Autodesk Inventor part; units mm, degrees
ref_plane "YZ Plane" through (0, 0, 0) normal (1, 0, 0) x (0, 1, 0)
ref_plane "XZ Plane" through (0, 0, 0) normal (0, 1, 0) x (-1, 0, 0)
ref_plane "XY Plane" through (0, 0, 0) normal (0, 0, 1) x (1, 0, 0)
sketch "Skizze1" plane through (0, 0, 0) normal (1, 0, 0) x (0, 1, 0)
  line L0 (-20, 20) -> (20, 20)
  line L1 (20, 20) -> (20, -20)
  line L2 (20, -20) -> (-20, -20)
  line L3 (-20, -20) -> (-20, 20)
  line L4 (-20, 20) -> (20, -20) construction
  line L5 (20, 20) -> (-20, -20) construction
  line L6 (-18, 18) -> (18, 18)
  line L7 (18, 18) -> (18, -18)
  line L8 (18, -18) -> (-18, -18)
  line L9 (-18, -18) -> (-18, 18)
  line L10 (-18, 18) -> (18, -18) construction
  line L11 (18, 18) -> (-18, -18) construction
  point P0 (0, 0)
  dimension "d0" = 40
  dimension "d1" = 40
  dimension "d2" = 36
  dimension "d3" = 36
extrude "Extrusion1" add sketch "Skizze1" along normal blind 1250
sketch "Skizze2" plane through (0, -20, 20) normal (0, 0, 1) x (1, 0, 0)
  circle A0 centre (20, 20) radius 5.25
  line L0 (1250, 2) -> (1250, 38)
  circle A1 centre (1150, 20) radius 5.25
  point P0 (0, 20)
  dimension "d7" = 10.5
  dimension "d11" = 10.5
extrude "Extrusion2" cut sketch "Skizze2" against normal blind 1250
sketch "Skizze3" plane through (0, 20, 20) normal (0, 1, 0) x (1, 0, 0)
  line L0 (0, 20) -> (110, 20)
  circle A0 centre (110, 20) radius 3.2
  dimension "d14" = 110
  dimension "d15" = 6.4
extrude "Extrusion3" cut sketch "Skizze3" against normal blind 5
sketch "Skizze4" plane through (0, -20, -20) normal (0, -1, 0) x (1, 0, 0)
  circle A0 centre (110, 20) radius 3.2
  line L0 (0, 20) -> (110, 20)
  circle A1 centre (110, 20) radius 5.5
  dimension "d18" = 110
  dimension "d19" = 11
extrude "Extrusion4" cut sketch "Skizze4" against normal blind 5 contours A0 | A1
fillet "Rundung1" radius 1 4 edges at (625, 20, -20) (625, -20, -20) (625, -20, 20) (625, 20, 20)
fillet "Rundung2" radius 0.5 4 edges at (625, -18, 18) (625, -18, -18) (625, 18, -18) (625, 18, 18)
sketch "Skizze6" plane through (0, -19, -20) normal (0, 0, -1) x (-1, 0, 0)
  line L0 (0, 19) -> (-500, 19)
  circle A0 centre (-500, 19) radius 14
  dimension "d28" = 500
  dimension "d29" = 28
extrude "Extrusion6" cut sketch "Skizze6" against normal blind 40
sketch "Skizze7" plane through (0, -19, 20) normal (0, 0, 1) x (1, 0, 0)
  line L0 (1250, 0) -> (1250, 38)
  line L1 (1250, 19) -> (1240, 19)
  circle A0 centre (1240, 19) radius 5.25
  point P0 (0, 19)
  dimension "d32" = 10
  dimension "d33" = 10.5
extrude "Extrusion7" cut sketch "Skizze7" against normal through all
properties part number "Längs_Traverse_hinten" material "Aluminium 6061"
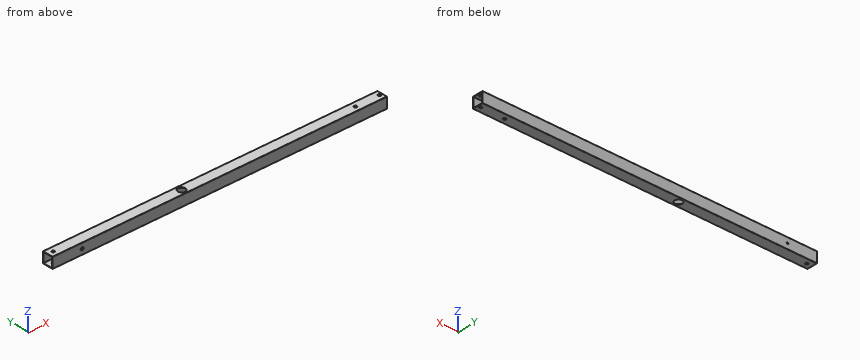
Source: CAD feature listing. Evaluate the final solid. Frame: model axes, mm. Give positions to 0.01 mm unless a question says otherwise; leave off trailing zeros. Loops run counter-clockwise (first coordinate to the right, second up) from the corner with the lowest first, then second, coordinate; pieces in that order, holes last. Notation, with made-up numbers: (-20, 38.25) - (26, 38.25) arc R15 cw to (26, 55.25) - close; hole circle Ø4 at (45.25, 45.25). An arc over 180 degrees is marked (long way). Use CSV: the item, a comma, the result in double quotes.
1) Cut plane B-B (x = 949.5). Output: boundary loops of the cut face in (y, z), and give its area (3 significant figures).
Worked out:
outline,"(-20, -19) arc R1 ccw to (-19, -20) - (19, -20) arc R1 ccw to (20, -19) - (20, 19) arc R1 ccw to (19, 20) - (-19, 20) arc R1 ccw to (-20, 19) - close; hole (-18, -17.5) arc R0.5 ccw to (-17.5, -18) - (17.5, -18) arc R0.5 ccw to (18, -17.5) - (18, 17.5) arc R0.5 ccw to (17.5, 18) - (-17.5, 18) arc R0.5 ccw to (-18, 17.5) - close"
area,"303 mm^2"
2) Line query: line 1 (Z direction, x = 837, y = 6). Output: solid intervals per line, ascending.
Worked out:
line 1,"z = -20 to -18, 18 to 20"
3) Pin query (flat end, axial travel): P1, Ø6.5, axis at x = 110, z = 0, coming from the -Y side; P2, Ø13.5, axis at x = 1240, y = 0, coming from the -Z side; P3, Ø9.5, axis at x = 1240, y = 0, coming from the +Z side. Return the tip coordinate at first contact, or that it passes through.
Worked out:
P1,"stops at y = 18"
P2,"stops at z = -20"
P3,"passes through"
4) Cut plane A-A (x = 500). Output: boundary loops of the cut face in (y, z), and give its area (3 significant figures).
Worked out:
outline,"(-20, -19) arc R1 ccw to (-19, -20) - (-14, -20) - (-14, -18) - (-17.5, -18) arc R0.5 cw to (-18, -17.5) - (-18, 17.5) arc R0.5 cw to (-17.5, 18) - (-14, 18) - (-14, 20) - (-19, 20) arc R1 ccw to (-20, 19) - close; (14, -20) - (19, -20) arc R1 ccw to (20, -19) - (20, 19) arc R1 ccw to (19, 20) - (14, 20) - (14, 18) - (17.5, 18) arc R0.5 cw to (18, 17.5) - (18, -17.5) arc R0.5 cw to (17.5, -18) - (14, -18) - close"
area,"191 mm^2"
